from build123d import *

# Parameters (mm, degrees)
F0_W     = 1270
F0_H     = 1270
F0_W_2   = 1016
F0_H_2   = 1016
F1_DEPTH = 635
F2_R     = 101.6
F3_SIZE  = 152.4
F4_DEPTH = 645.067396


with BuildPart() as f1:
    # F0 (on Front) → F1 (new body, symmetric)
    with BuildSketch(Plane.XZ):
        Rectangle(F0_W, F0_H)
        Rectangle(F0_W_2, F0_H_2, mode=Mode.SUBTRACT)
    extrude(amount=F1_DEPTH, both=True)

    # F2
    f2_edges = [f1.edges().sort_by_distance(p)[0] for p in [
        (635, 0, 635),
    ]]
    fillet(f2_edges, radius=F2_R)

    # F3
    f3_edges = [f1.edges().sort_by_distance(p)[0] for p in [
        (-508, 0, -508),
    ]]
    chamfer(f3_edges, length=F3_SIZE)

    # F1_face (on face) → F4 (join)
    with BuildSketch(Plane(origin=(-11.297191, -635, -11.297191), x_dir=(1, 0, 0), z_dir=(0, -1, 0))):
        with BuildLine():
            Line((646.297191, -623.702809), (646.297191, 544.697191))
            ThreePointArc((646.297191, 544.697191), (616.53924, 616.53924), (544.697191, 646.297191))
            Line((544.697191, 646.297191), (-623.702809, 646.297191))
            Line((-623.702809, 646.297191), (-623.702809, -623.702809))
            Line((-623.702809, -623.702809), (646.297191, -623.702809))
        make_face()
        Polygon((519.297191, -496.702809), (-344.302809, -496.702809), (-496.702809, -344.302809), (-496.702809, 519.297191), (519.297191, 519.297191), align=None, mode=Mode.SUBTRACT)
    extrude(amount=F4_DEPTH)


solid = f1.part
Read the model definition and answer for the solid it produces. Units are mm, in the model's axes. A direction names the side the tool comes from. Give positions to 0.01 mm unless a question says otherwise; leave off trailing zeros. Write each loop counter-clockwise with the first axis right and the second up, starting at its lowest first coordinate (ties: lowest second). Pieces come first, ordered by that corner, then holes. Notation, with made-up numbers: (-30, 58.25) -> (1, 58.25) arc R21 cw to (1, 83.25) -> close; hole circle Ø3 at (23.25, 45). An arc over 180 degrees is marked (long way). Answer as a JSON object with one key per item and string values. Group by question number.
1) The mould has two halves that part along Z. Classify faces 1 (the flat face through (-508, -309, 70)), 2 (the flat face through (-43, -309, 635)), 3 (the flat face through (-573, -1280.067, 9)): +Z half, -Z half, draft (parallel to the pull), parting line (faces both ways), or undercut.
2) A tool of negligible diameter and unlimited length cuts with its end or side. For faces 4 (the flat face through (-430.7, -309.1, -432.9)), 5 (the flat face through (635, -309, -59)), from which of +Z, -Z, +X, -X, +Y, -Y can it reach the whole face along a straight path? Write none if from no direction.
3) Consider L1, parallel to X at y = -1111, z = 101.5; L2, parallel to Z at x = -356.5, y = 550. Determine where each line is inside the solid, lowest interval first. Write a range as from..to.
4) Find section C-C (y = 162). Write down the section's boundary in (x, z).
5) Find section B-B (x = -406). Write down the section's boundary in (y, z).
6) Find section A-A (z = -444). Write down the section's boundary in (x, y).
Values follow:
{
 "1": {"face 1": "undercut", "face 2": "+Z half", "face 3": "draft"},
 "2": {"face 4": "+Y, -Y", "face 5": "+Z, -Z, +X, +Y, -Y"},
 "3": {"L1": "x = -635..-508, 508..635", "L2": "z = -635..-507.1, 508..635"},
 "4": {"outline": "(-635, -635) -> (635, -635) -> (635, 533.4) arc R101.6 ccw to (533.4, 635) -> (-635, 635) -> close; hole (-508, -355.6) -> (-355.6, -508) -> (508, -508) -> (508, 508) -> (-508, 508) -> close"},
 "5": {"outline": "(-1280.07, -635) -> (635, -635) -> (635, -457.6) -> (-1280.07, -457.6) -> close; (-1280.07, 508) -> (635, 508) -> (635, 635) -> (-1280.07, 635) -> close"},
 "6": {"outline": "(-635, -1280.07) -> (-419.6, -1280.07) -> (-419.6, 635) -> (-635, 635) -> close; (508, -1280.07) -> (635, -1280.07) -> (635, 635) -> (508, 635) -> close"}
}
